CAD build for the part. Positions are in the model's coordinates, mm. A direction names the side the tool comes from. Round coordinates to 2 decimals unless told otherwise and drop trailing zeros. Loops run counter-clockwise (first coordinate to the right, second up) from the corner with the lowest first, then second, coordinate; pieces in that order, holes last.
Autodesk Inventor part; units mm, degrees
ref_plane "YZ Plane" through (0, 0, 0) normal (1, 0, 0) x (0, 1, 0)
ref_plane "XZ Plane" through (0, 0, 0) normal (0, 1, 0) x (-1, 0, 0)
ref_plane "XY Plane" through (0, 0, 0) normal (0, 0, 1) x (1, 0, 0)
sketch "Boceto1" plane through (0, 0, 0) normal (0, 1, 0) x (-1, 0, 0)
  arc A0 (117.4998, -25.6738) -> (124.3299, -32.5039) centre (119.9998, -30.0039) ccw
  circle A1 centre (119.9998, -30.0039) radius 1.5
  line L0 (119.9998, -12.5039) -> (119.9998, -21.3437)
  arc A2 (117.4998, -25.6738) -> (119.9998, -21.3437) centre (114.9998, -21.3437) ccw
  arc A3 (128.66, -30.0039) -> (124.3299, -32.5039) centre (128.66, -35.0039) ccw
  arc A4 (118.7343, 12.4319) -> (119.9998, -12.5039) centre (119.9994, -0.0039) ccw
  line L1 (133.4998, 22.4961) -> (121.2045, 13.3885)
  line L2 (164.9248, 22.4961) -> (164.9248, -25.0039)
  line L3 (159.9248, -30.0039) -> (128.66, -30.0039)
  line L4 (164.9248, 22.4961) -> (133.4998, 22.4961)
  line L5 (149.2123, 17.4961) -> (144.2123, 17.4961)
  line L6 (144.2123, 17.4961) -> (144.2123, 14.4961)
  line L7 (144.2123, 14.4961) -> (154.2123, 14.4961)
  line L8 (154.2123, 14.4961) -> (154.2123, 17.4961)
  line L9 (154.2123, 17.4961) -> (149.2123, 17.4961)
  line L10 (149.2123, 6.4961) -> (144.2123, 6.4961)
  line L11 (144.2123, 6.4961) -> (144.2123, 3.4961)
  line L12 (144.2123, 3.4961) -> (154.2123, 3.4961)
  line L13 (154.2123, 3.4961) -> (154.2123, 6.4961)
  line L14 (154.2123, 6.4961) -> (149.2123, 6.4961)
  line L15 (160.0685, -12.0039) -> (160.0685, -15.0039)
  circle A5 centre (119.9994, -0.0039) radius 1.5
  line L16 (160.0685, -12.0039) -> (152.0685, -12.0039)
  line L17 (152.0685, -12.0039) -> (152.0685, -15.0039)
  line L18 (152.0685, -15.0039) -> (160.0685, -15.0039)
  line L19 (146.0685, -12.0039) -> (146.0685, -15.0039)
  line L20 (146.0685, -15.0039) -> (138.0685, -15.0039)
  line L21 (138.0685, -15.0039) -> (138.0685, -12.0039)
  line L22 (132.0685, -12.0039) -> (132.0685, -15.0039)
  line L23 (132.0685, -15.0039) -> (126.0685, -15.0039)
  line L24 (126.0685, -15.0039) -> (126.0685, -12.0039)
  line L25 (126.0685, -12.0039) -> (132.0685, -12.0039)
  line L26 (138.0685, -12.0039) -> (146.0685, -12.0039)
  arc A6 (159.9248, -30.0039) -> (164.9248, -25.0039) centre (159.9248, -25.0039) ccw
  arc A7 (118.7343, 12.4319) -> (121.2045, 13.3885) centre (118.2283, 17.4062) ccw
  point P0 (124.9998, -30.0039)
  point P1 (119.9998, -25.0039)
  point P2 (119.9998, 12.4961)
  dimension "d165" = 8
  dimension "d166" = 6
  dimension "d167" = 8
  dimension "d169" = 6
  dimension "d170" = 5
extrude "Extrusión1" add sketch "Boceto1" along normal blind 3
properties part number "codo"
Item 1: Wall check: L1, parallel to X at y = 1.6, z = -14.5; L2, parallel to Z at x = -158.5, y = 1.5; L3, parallel to X at y = 1.65, z = -20.5. Give the ranges that are in metal, low to high.
Verdict:
L1: x = -164.92 to -160.07, -152.07 to -146.07, -138.07 to -132.07, -126.07 to -120
L2: z = -30 to -15, -12 to 22.5
L3: x = -164.92 to -120
Item 2: Cut at A-A (x = -149). List the corners of the cut face in (y, z), plus the area to 4 significant figures.
Verdict:
outline: (0, -30) - (3, -30) - (3, 3.5) - (0, 3.5) - close; (0, 6.5) - (3, 6.5) - (3, 14.5) - (0, 14.5) - close; (0, 17.5) - (3, 17.5) - (3, 22.5) - (0, 22.5) - close
area: 139.5 mm2
Item 3: Cut at D-D (z = -17). List the corners of the cut face in (x, y), plus the area to 3 significant figures.
Verdict:
outline: (-164.92, 0) - (-120, 0) - (-120, 3) - (-164.92, 3) - close
area: 135 mm2
Item 4: 3-axis set-ups, long thin cutter, end or side, ignore diameter. For faces 5 (the cylindrical face through (-107.53, 1.48, -0.9)), 6 (the flat face through (-156, 1, -12.004)): which of +Z, -Z, +X, -X, +Y, -Y reach the whole face in a straight line?
Verdict:
face 5: +X, +Y, -Y
face 6: +Y, -Y
Item 5: Cut at C-C (y = 1.1). State how many separate pieces and enclosed holes the cut face has, plus the area to 3 significant figures.
Verdict:
separate pieces: 1
enclosed holes: 7
area: 2,450 mm2
Item 6: Flat gauge pins, fed straight in: P1, Ø0.9, axis at x = -128, y = 2, coming from the -Z side; P2, Ø1.5, axis at x = -143, y = 1.5, coming from the -Z side; P3, Ø0.9, axis at y = 1.5, z = -14, coming from the +X side. Where does each tip first touch, or does it go through?
Verdict:
P1: stops at z = -30.13
P2: stops at z = -30
P3: stops at x = -120
Item 7: Mould opens along Z. For faces 1 (the flat face through (-145, 1, -30.004)), 2 (the flat face through (-152.068, 1, -13)), 3 (the flat face through (-149, 1, 22.496)), 4 (the flat face through (-138.068, 1, -14)) say: released by +Z, released by -Z, zero draft, split by the parting line, or undercut.
Verdict:
face 1: released by -Z
face 2: undercut
face 3: released by +Z
face 4: undercut
Item 8: Cut at B-B (x = -155). List the corners of the cut face in (y, z).
Verdict:
outline: (0, -30) - (3, -30) - (3, -15) - (0, -15) - close; (0, -12) - (3, -12) - (3, 22.5) - (0, 22.5) - close
